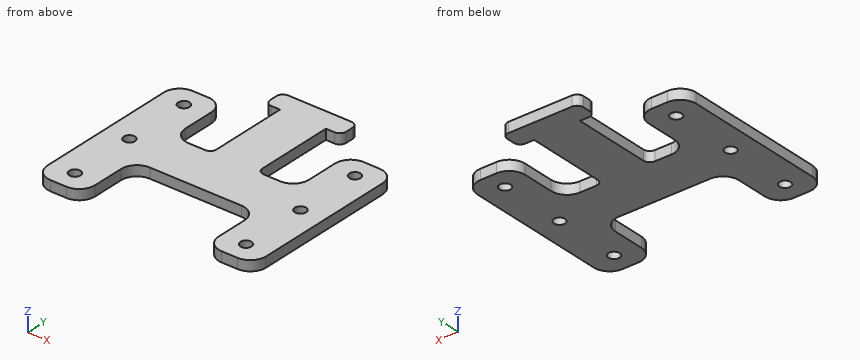
from build123d import *

# Parameters (mm, degrees)
F0_R     = 1.778
F1_DEPTH = 3.2


with BuildPart() as f1:
    # F0 (on Top) → F1 (new body)
    with BuildSketch(Plane.XY):
        with BuildLine():
            ThreePointArc((0, 5), (1.464466, 1.464466), (5, 0))
            Line((5, 0), (10, 0))
            ThreePointArc((10, 0), (13.535534, 1.464466), (15, 5))
            Line((15, 5), (15, 15))
            ThreePointArc((15, 15), (16.464466, 18.535534), (20, 20))
            Line((20, 20), (34.455914, 20))
            Line((34.455914, 20), (48.911828, 20))
            ThreePointArc((48.911828, 20), (52.447362, 18.535534), (53.911828, 15))
            Line((53.911828, 15), (53.911828, 5))
            ThreePointArc((53.911828, 5), (55.376294, 1.464466), (58.911828, 0))
            Line((58.911828, 0), (63.911828, 0))
            ThreePointArc((63.911828, 0), (67.447362, 1.464466), (68.911828, 5))
            Line((68.911828, 5), (68.911828, 50))
            ThreePointArc((68.911828, 50), (67.447362, 53.535534), (63.911828, 55))
            Line((63.911828, 55), (58.911828, 55))
            ThreePointArc((58.911828, 55), (55.376294, 53.535534), (53.911828, 50))
            Line((53.911828, 50), (53.911828, 40))
            ThreePointArc((53.911828, 40), (52.447362, 36.464466), (48.911828, 35))
            Line((48.911828, 35), (43.683871, 35))
            ThreePointArc((43.683871, 35), (42.269658, 35.585786), (41.683871, 37))
            Line((41.683871, 37), (41.683871, 61.580155))
            Line((41.683871, 61.580155), (44.441202, 61.580155))
            ThreePointArc((44.441202, 61.580155), (45.855415, 62.165942), (46.441202, 63.580155))
            Line((46.441202, 63.580155), (46.441202, 66.080155))
            ThreePointArc((46.441202, 66.080155), (45.855415, 67.494369), (44.441202, 68.080155))
            Line((44.441202, 68.080155), (34.455914, 68.080155))
            Line((34.455914, 68.080155), (24.470626, 68.080155))
            ThreePointArc((24.470626, 68.080155), (23.056413, 67.494369), (22.470626, 66.080155))
            Line((22.470626, 66.080155), (22.470626, 63.580155))
            ThreePointArc((22.470626, 63.580155), (23.056413, 62.165942), (24.470626, 61.580155))
            Line((24.470626, 61.580155), (27.227957, 61.580155))
            Line((27.227957, 61.580155), (27.227957, 37))
            ThreePointArc((27.227957, 37), (26.642171, 35.585786), (25.227957, 35))
            Line((25.227957, 35), (20, 35))
            ThreePointArc((20, 35), (16.464466, 36.464466), (15, 40))
            Line((15, 40), (15, 50))
            ThreePointArc((15, 50), (13.535534, 53.535534), (10, 55))
            Line((10, 55), (5, 55))
            ThreePointArc((5, 55), (1.464466, 53.535534), (0, 50))
            Line((0, 50), (0, 5))
        make_face()
        with Locations((7.5, 6.380155)):
            Circle(F0_R, mode=Mode.SUBTRACT)
        with Locations((7.5, 27.480155)):
            Circle(F0_R, mode=Mode.SUBTRACT)
        with Locations((61.411828, 6.380155)):
            Circle(F0_R, mode=Mode.SUBTRACT)
        with Locations((61.411828, 27.480155)):
            Circle(F0_R, mode=Mode.SUBTRACT)
        with Locations((7.5, 48.580155)):
            Circle(F0_R, mode=Mode.SUBTRACT)
        with Locations((61.411828, 48.580155)):
            Circle(F0_R, mode=Mode.SUBTRACT)
    extrude(amount=F1_DEPTH)


solid = f1.part
Could you check a few things on this model? Use its own coordinates, in mm. Coordinates: 2 decimals unless noted, no trailing zeros. Write each loop counter-clockwise with the first axis right and the second up, starting at its lowest first coordinate (ties: lowest second). Pieces come first, ordered by that corner, then holes. Notation, with made-up numbers: M 81,-30.75 L 125,-30.75 A27 cw 125,-10.75 Z; hole C -34,-7 d1. An arc over 180 degrees is marked long. One line per question, with ' | ' between items.
1) Imagine slicing it at D-D, the plane x = 36. Write out the boundary of the cut face in (y, z).
Checks:
outline: M 20,0 L 68.08,0 L 68.08,3.2 L 20,3.2 Z
2) Imagine slicing it at C-C, the plane z = 0.7. Give the number of separate pieces and of enclosed holes in the cut face, and give its area (3 significant figures).
Checks:
separate pieces: 1 | enclosed holes: 6 | area: 2,690 mm²
3) For pin 1 Ø1 at (x, z) = (6.5, 1) entering from +Y; pin 2 Ø3 at (x, y) = (7.5, 27.48) entering from +Z; pin 3 Ø1.6 at (x, z) = (45, 1.5) entering from +Y; pin 4 Ø0.8 at (x, z) = (25.5, 2) entering from -Y, each with a flat end and sliding along its axis, tell me the tip position at first contact or that it passes through.
Checks:
pin 1: y = 55 | pin 2: through | pin 3: y = 68.08 | pin 4: y = 20
4) Imagine slicing it at B-B, the plane y = 26.5. Write out the boundary of the cut face in (x, z).
Checks:
outline: M 0,0 L 6.02,0 L 6.02,3.2 L 0,3.2 Z; M 8.98,0 L 59.93,0 L 59.93,3.2 L 8.98,3.2 Z; M 62.9,0 L 68.91,0 L 68.91,3.2 L 62.9,3.2 Z
5) I need wall thicknesses on probe 1 along Y at (x, z) = (7.5, 1.85); probe 2 along X at (y, z) = (46.5, 1.6); probe 3 along X at (y, z) = (5, 0.55). Which ranges of each line are inside material? Lowest first, please. Write a range as [from, to].
Checks:
probe 1: [0, 4.6], [8.16, 25.7], [29.26, 46.8], [50.36, 55] | probe 2: [0, 15], [27.23, 41.68], [53.91, 68.91] | probe 3: [0, 6.38], [8.62, 15], [53.91, 60.29], [62.53, 68.91]
6) Imagine slicing it at A-A, the plane x = 7.5. Write out the boundary of the cut face in (y, z).
Checks:
outline: M 0,0 L 4.6,0 L 4.6,3.2 L 0,3.2 Z; M 8.16,0 L 25.7,0 L 25.7,3.2 L 8.16,3.2 Z; M 29.26,0 L 46.8,0 L 46.8,3.2 L 29.26,3.2 Z; M 50.36,0 L 55,0 L 55,3.2 L 50.36,3.2 Z
